from build123d import *

# Parameters (mm, degrees)
ESQUISSE1_R             = 105
ESQUISSE1_R_2           = 4
BOSS_EXTRU_1_DEPTH      = 5
ESQUISSE2_W             = 250
ESQUISSE2_H             = 50
ENL_V_MAT_EXTRU_1_DEPTH = 149.576579581


with BuildPart() as part:
    # Esquisse1 → Boss.-Extru.1 (new body)
    with BuildSketch(Plane.XY):
        Circle(ESQUISSE1_R)
        with Locations((-80, 50)):
            Circle(ESQUISSE1_R_2, mode=Mode.SUBTRACT)
        with Locations(Location((80, 50, 0), (0, 0, 180))):
            Circle(ESQUISSE1_R_2, mode=Mode.SUBTRACT)
        with Locations((80, -50)):
            Circle(ESQUISSE1_R_2, mode=Mode.SUBTRACT)
        with Locations(Location((-80, -50, 0), (0, 0, 180))):
            Circle(ESQUISSE1_R_2, mode=Mode.SUBTRACT)
    extrude(amount=BOSS_EXTRU_1_DEPTH)

    # Esquisse2 → Enlèv. mat.-Extru.1 (cut, through all)
    with BuildSketch(Plane.XY.offset(5)):
        with Locations((0, 85)):
            Rectangle(ESQUISSE2_W, ESQUISSE2_H)
        with Locations((0, -85)):
            Rectangle(ESQUISSE2_W, ESQUISSE2_H)
    extrude(amount=-ENL_V_MAT_EXTRU_1_DEPTH, mode=Mode.SUBTRACT)


solid = part.part
Could you check a few things on this model? Use its own coordinates, in mm. Give positions to 0.01 mm unless a question says otherwise; leave off trailing zeros. Order: outer loops, then holes, each group sorted by start corner. A loop starts at its lowest first (then second) coordinate and runs counter-clockwise, first axis right, second up.
1. Thinking about a two-plate mould opening in Y: for faces 1 (the cylindrical face through (83.695, -51.532, 2.465)), 2 (the flat face through (-1, 1, 0)), 3 (the flat face through (-1, 60, 3)), which applies, +Y half, -Y half, draft (parallel to the pull), parting line (faces both ways), or undercut?
Answers below:
face 1: undercut
face 2: draft
face 3: +Y half
2. Suppose I cut it at B-B (z = 3.75). Write out the boundary of the cut face in (x, y), plus the area to 3 significant figures.
Answers below:
outline: (-86.17, -60) - (86.17, -60) arc R105 ccw to (86.17, 60) - (-86.17, 60) arc R105 ccw to start; hole circle Ø8 at (-80, -50); hole circle Ø8 at (-80, 50); hole circle Ø8 at (80, -50); hole circle Ø8 at (80, 50)
area: 23,600 mm2
3. For pin 1 (5 mm diameter, centred on x = 80, y = -50, fed in from -Z); pin 2 (1 mm diameter, centred on y = 30.5, z = 3.5, fed in from +X), each with a flat end and sliding along its axis, tell me the tip position at first contact or that it passes through.
Answers below:
pin 1: passes through
pin 2: stops at x = 100.62
4. I need wall thicknesses on L1, parallel to Y at x = -80, z = 3; L2, parallel to Y at x = 81, z = 1.1; L3, parallel to X at y = 48, z = 1.7. Which ranges of each line are inside material? Lowest first, please.
Answers below:
L1: y = -60 to -54, -46 to 46, 54 to 60
L2: y = -60 to -53.87, -46.13 to 46.13, 53.87 to 60
L3: x = -93.39 to -83.46, -76.54 to 76.54, 83.46 to 93.39
5. Suppose I cut it at A-A (x = -80). Write out the boundary of the cut face in (y, z).
Answers below:
outline: (-60, 0) - (-54, 0) - (-54, 5) - (-60, 5) - close; (-46, 0) - (46, 0) - (46, 5) - (-46, 5) - close; (54, 0) - (60, 0) - (60, 5) - (54, 5) - close
6. Suppose I cut it at D-D (y = -28). Write out the boundary of the cut face in (x, z).
Answers below:
outline: (-101.2, 0) - (101.2, 0) - (101.2, 5) - (-101.2, 5) - close
7. Suppose I cut it at C-C (y = -50). Write out the boundary of the cut face in (x, z), plus the area to 3 significant figures.
Answers below:
outline: (-92.33, 0) - (-84, 0) - (-84, 5) - (-92.33, 5) - close; (-76, 0) - (76, 0) - (76, 5) - (-76, 5) - close; (84, 0) - (92.33, 0) - (92.33, 5) - (84, 5) - close
area: 843 mm2
